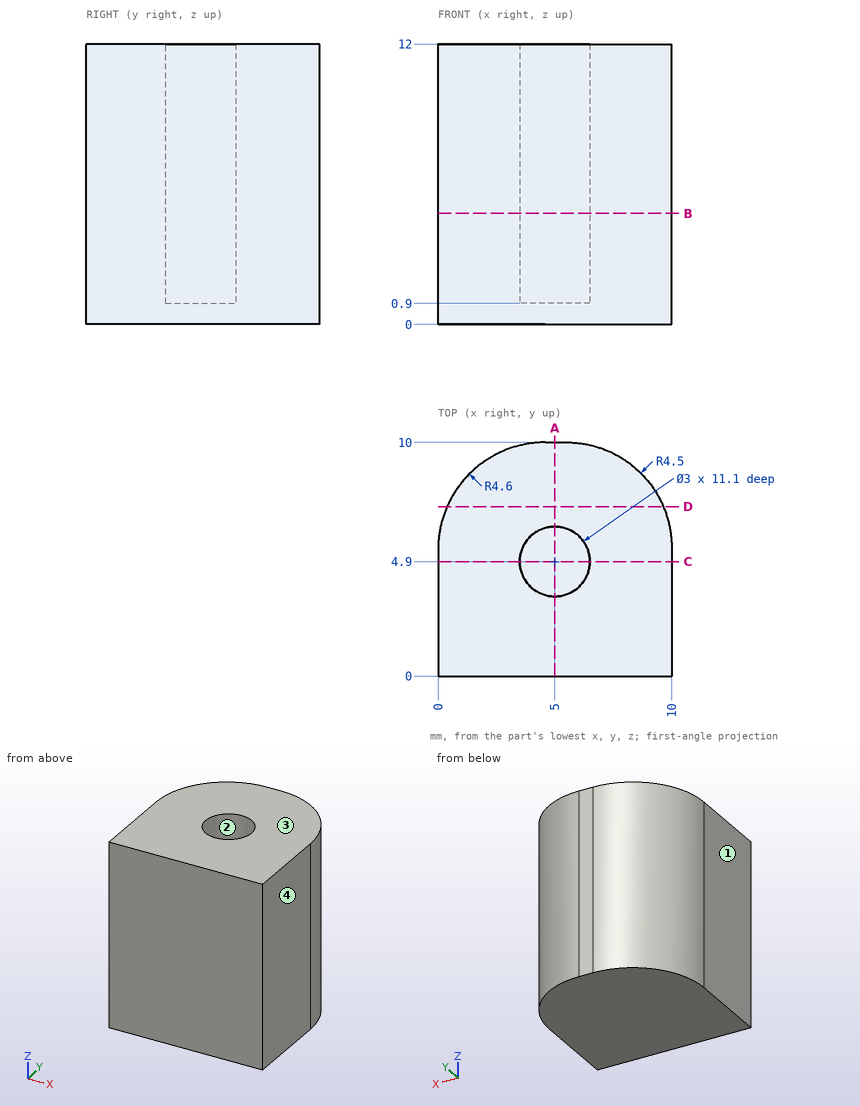
Could you check a few things on this drawing? It's one solid part, dimensions in mm from its lowest x, y, z. Give positions to 0.01 mm unless a question says otherwise; leave off trailing zeros. Order: outer loops, then holes, each group sorted by start corner. A loop starts at its lowest first (then second) coordinate and runs counter-clockwise, first axis right, second up. Notation, with made-up numbers: M 17,29.25 L 67,29.25 A17 cw 67,49.25 Z; hole C -9,67.5 d11. An arc over 180 degrees is marked long. Use one line per item in the form item = value. Start each with the question number.
Item 1: If we section it at C-C (y = 4.9): Write out the boundary of the cut face in (x, z), then the cut area to 3 significant figures.
Item 2: If we section it at B-B (z = 4.75): Write out the boundary of the cut face in (x, y).
Item 3: If we section it at D-D (y = 7.25): Write out the boundary of the cut face in (x, z).
Item 4: We'd pull the mould along X, two halves only. Please class the marked faces 1, 2, 3 and 4: +X half, -X half, draft (parallel to the pull), parting line (faces both ways), or undercut.
Item 5: If we section it at A-A (x = 5): Write out the boundary of the cut face in (y, z), then the cut area to 3 significant figures.
Item 6: If I drill on line 1 along X through (y, z) = (4.9, 6.5); line 2 along Y through (x, z) = (5.25, 2.5); line 3 along Y through (x, z) = (2.5, 1.75), over which ranges is the centre line in solid material (lowest first)?
Item 7: Will this pin go through, and if not, where does the flat tip stop? pin 1 Ø5 at (x, y) = (1.5, 8) entering from -Z.
Outcome:
q1.outline = M 0,0 L 10,0 L 10,12 L 6.5,12 L 6.5,0.9 L 3.5,0.9 L 3.5,12 L 0,12 Z
q1.area = 86.7 mm2
q2.outline = M 0,0 L 10,0 L 10,5.5 A4.5 ccw 5.5,10 L 4.6,10 A4.6 ccw 0,5.4 Z; hole C 5,4.9 d3
q3.outline = M 0.39,0 L 9.65,0 L 9.65,12 L 0.39,12 Z
q4.face_1 = -X half
q4.face_2 = undercut
q4.face_3 = draft
q4.face_4 = +X half
q5.outline = M 0,0 L 10,0 L 10,12 L 6.4,12 L 6.4,0.9 L 3.4,0.9 L 3.4,12 L 0,12 Z
q5.area = 86.7 mm2
q6.line_1 = 0 to 3.5, 6.5 to 10
q6.line_2 = 0 to 3.42, 6.38 to 10
q6.line_3 = 0 to 9.49
q7.pin_1 = 0
